from build123d import *

# Parameters (mm, degrees)
EXTRUDE_1_DEPTH          = 40
SKETCH_2_R               = 13
CUT_EXTRUDE_1_DEPTH      = 1.5
SKETCH_3_R               = 13
CUT_EXTRUDE_2_DEPTH      = 50.862310416
CUT_EXTRUDE_3_REACH      = 52.319
SKETCH_4_R               = 2
PATTERN_CIRCULAR_1_COUNT = 4
SKETCH_5_R               = 1.5
CUT_EXTRUDE_4_DEPTH      = 49.744230428
SKETCH_6_W               = 33
SKETCH_6_H               = 40
CUT_EXTRUDE_5_DEPTH      = 1.5
SKETCH_7_W               = 6
SKETCH_7_H               = 40
CUT_EXTRUDE_6_DEPTH      = 2
EXTRUDE_2_DEPTH          = 5
SKETCH_9_W               = 33
SKETCH_9_H               = 4
EXTRUDE_3_DEPTH          = 12.5
SKETCH_10_R              = 1.6
CUT_EXTRUDE_7_DEPTH      = 4
CUT_EXTRUDE_START        = -3
SKETCH_11_R              = 3
SKETCH_11_R_2            = 1.6
CUT_EXTRUDE_8_DEPTH      = 3
SKETCH_12_R              = 3
CUT_EXTRUDE_9_DEPTH      = 14


with BuildPart() as part:
    # 草图1 → 凸台-拉伸1 (new body)
    with BuildSketch(Plane.XY):
        Polygon((-16.5, 27.398785639), (-16.5, 16.398785639), (16.5, 16.398785639), (16.5, 27.398785639), (26, 27.398785639), (26, 21.398785639), (20, 21.398785639), (20, 16.398785639), (20, 11.398785639), (-20, 11.398785639), (-20, 21.398785639), (-26, 21.398785639), (-26, 27.398785639), align=None)
    extrude(amount=EXTRUDE_1_DEPTH)

    # 草图2 → 切除-拉伸1 (cut)
    with BuildSketch(Plane.XZ.offset(-11.398785639)):
        with Locations(Location((0, 20, 0), (0, 0, 270))):
            Circle(SKETCH_2_R)
    extrude(amount=-CUT_EXTRUDE_1_DEPTH, mode=Mode.SUBTRACT)

    # 草图3 → 切除-拉伸2 (cut, through all)
    with BuildSketch(Plane.XZ.offset(-12.898785639)):
        with Locations(Location((0, 20, 0), (0, 0, 270))):
            Circle(SKETCH_3_R)
    extrude(amount=-CUT_EXTRUDE_2_DEPTH, mode=Mode.SUBTRACT)

    # 草图4 → 切除-拉伸3 (cut, up to next)
    with BuildSketch(Plane.XZ.offset(-11.398785639), mode=Mode.PRIVATE) as cut_extrude_3_sk1:
        with Locations(Location((12.374368671, 32.374368671, 0), (0, 0, 270))):
            Circle(SKETCH_4_R)
    cut_extrude_3_tool1 = extrude(cut_extrude_3_sk1.sketch, amount=-CUT_EXTRUDE_3_REACH, mode=Mode.PRIVATE) & part.part
    cut_extrude_3 = cut_extrude_3_tool1.solids().sort_by_distance((12.374369, 11.398786, 32.374369))[0]
    add(cut_extrude_3, mode=Mode.SUBTRACT)

    # 阵列(圆周)1: 切除-拉伸3 ×4 about axis
    pattern_circular_1_axis = Axis((0, 0, 20), (0, 1, 0))
    for i in range(1, PATTERN_CIRCULAR_1_COUNT):
        add(cut_extrude_3.rotate(pattern_circular_1_axis, i * 360 / PATTERN_CIRCULAR_1_COUNT), mode=Mode.SUBTRACT)

    # 草图5 → 切除-拉伸4 (cut, through all)
    with BuildSketch(Plane.XZ.offset(-21.398785639)):
        with Locations(Location((-23, 27.5, 0), (0, 0, 270))):
            Circle(SKETCH_5_R)
        with Locations(Location((-23, 12.5, 0), (0, 0, 270))):
            Circle(SKETCH_5_R)
    cut_extrude_4 = extrude(amount=-CUT_EXTRUDE_4_DEPTH, mode=Mode.SUBTRACT)

    # 镜向1: 切除-拉伸4 across plane
    add(cut_extrude_4.mirror(Plane.ZY), mode=Mode.SUBTRACT)

    # 草图6 → 切除-拉伸5 (cut)
    with BuildSketch(Plane(origin=(0, 16.398785639, 0), x_dir=(1, 0, 0), z_dir=(0, 1, 0))):
        with Locations((0, -20)):
            Rectangle(SKETCH_6_W, SKETCH_6_H)
    extrude(amount=-CUT_EXTRUDE_5_DEPTH, mode=Mode.SUBTRACT)

    # 草图7 → 切除-拉伸6 (cut)
    with BuildSketch(Plane.XZ.offset(-21.398785639)):
        with Locations((-23, 20)):
            Rectangle(SKETCH_7_W, SKETCH_7_H)
        with Locations((23, 20)):
            Rectangle(SKETCH_7_W, SKETCH_7_H)
    extrude(amount=-CUT_EXTRUDE_6_DEPTH, mode=Mode.SUBTRACT)

    # 草图8 → 凸台-拉伸2 (add)
    with BuildSketch(Plane.XY):
        Polygon((20, 11.398785639), (20, 23.398785639), (26, 23.398785639), (26, 27.398785639), (16.5, 27.398785639), (16.5, 14.898785639), (-16.5, 14.898785639), (-16.5, 27.398785639), (-26, 27.398785639), (-26, 23.398785639), (-20, 23.398785639), (-20, 11.398785639), align=None)
    extrude(amount=-EXTRUDE_2_DEPTH)

    # 草图9 → 凸台-拉伸3 (add)
    with BuildSketch(Plane(origin=(0, 14.898785639, 0), x_dir=(1, 0, 0), z_dir=(0, 1, 0))):
        with Locations((0, 3)):
            Rectangle(SKETCH_9_W, SKETCH_9_H)
    extrude(amount=EXTRUDE_3_DEPTH)

    # 草图10 → 切除-拉伸7 (cut)
    with BuildSketch(Plane(origin=(0, 0, -5), x_dir=(-1, 0, 0), z_dir=(0, 0, -1))):
        with Locations((-11, 23.398785639)):
            Circle(SKETCH_10_R)
        with Locations((0, 17.398785639)):
            Circle(SKETCH_10_R)
        with Locations((11, 23.398785639)):
            Circle(SKETCH_10_R)
    extrude(amount=-CUT_EXTRUDE_7_DEPTH, mode=Mode.SUBTRACT)

    # 草图11 → 切除-拉伸8 (cut)
    # profile 1 of 3: a face of its own
    with BuildSketch(Plane.XY.offset(-1).offset(CUT_EXTRUDE_START)):
        with Locations((-11, 23.398785639)):
            Circle(SKETCH_11_R)
        with Locations(Location((-11, 23.398785639, 0), (0, 0, 180))):
            Circle(SKETCH_11_R_2, mode=Mode.SUBTRACT)
    # profile 2 of 3: a face of its own
    with BuildSketch(Plane.XY.offset(-1).offset(CUT_EXTRUDE_START)):
        with Locations((0, 17.398785639)):
            Circle(SKETCH_11_R)
        with Locations(Location((0, 17.398785639, 0), (0, 0, 180))):
            Circle(SKETCH_11_R_2, mode=Mode.SUBTRACT)
    # profile 3 of 3: a face of its own
    with BuildSketch(Plane.XY.offset(-1).offset(CUT_EXTRUDE_START)):
        with Locations((11, 23.398785639)):
            Circle(SKETCH_11_R)
        with Locations(Location((11, 23.398785639, 0), (0, 0, 180))):
            Circle(SKETCH_11_R_2, mode=Mode.SUBTRACT)
    extrude(amount=CUT_EXTRUDE_8_DEPTH, mode=Mode.SUBTRACT)

    # 草图12 → 切除-拉伸9 (cut)
    with BuildSketch(Plane.XY.offset(-1)):
        with Locations((0, 17.398785639)):
            Circle(SKETCH_12_R)
    extrude(amount=CUT_EXTRUDE_9_DEPTH, mode=Mode.SUBTRACT)


solid = part.part
Input: part model. Units: mm. Frame: model coordinates. A direction names the side the tool comes from. Give positions to 0.01 mm unless a question says otherwise; leave off trailing zeros. Write each loop counter-clockwise with the first axis right and the second up, starting at its lowest first coordinate (ties: lowest second). Pieces come first, ordered by that corner, then holes. Notation, with made-up numbers: M 2.5,49.5 L 53.5,49.5 A35 cw 53.5,83.5 Z; hole C 25,63 d1. An arc over 180 degrees is marked long. Use one line per item in the form item = value.
1. Reachability of faces 1 (the face through (12.3, 22.1, -4)), 2 (the face through (20, 17, 18)), 3 (the face through (-20, 17, 18)), 4 (the face through (-16.5, 21, 20)) from +Z, -Z, +X, -X, +Y, -Y: full face, straight path, thin tool, end or side. Return the list, or none.
Outcome:
face_1 = +Z
face_2 = +Z, -Z, +X, -Y
face_3 = +Z, -Z, -X, -Y
face_4 = +Z, +Y
2. Cut plane A-A on z = 20. Return loops of the section in (x, y), and give its area (4 significant figures).
Outcome:
outline = M -26,23.4 L -20,23.4 L -20,11.4 L -13,11.4 L -13,14.9 L -16.5,14.9 L -16.5,27.4 L -26,27.4 Z; M 13,11.4 L 20,11.4 L 20,23.4 L 26,23.4 L 26,27.4 L 16.5,27.4 L 16.5,14.9 L 13,14.9 Z
area = 184.5 mm²
3. Ray query, L1, parallel to X at y = 25.8, z = 27.5; L2, parallel to X at y = 26.5, z = 22; L3, parallel to X at y = 15.25, z = 12. Return the intervals inside material, ascending.
Outcome:
L1 = -26 to -24.5, -21.5 to -16.5, 16.5 to 21.5, 24.5 to 26
L2 = -26 to -16.5, 16.5 to 26
L3 = -20 to -16.5, 16.5 to 20
4. Mould query, pull axis Y, two halves, no side actions, for faces 5 (the face through (0, 27.399, -3)), 6 (the face through (8.6, 21.6, -2.5)), 7 (the face through (0, 21, -1)). Classes: released by +Y, released by -Y, zero draft, split by the parting line, or undercut.
Outcome:
face_5 = released by +Y
face_6 = undercut
face_7 = zero draft
5. Cut plane B-B on x = 23. Return loops of the section in (y, z), and give its area (3 significant figures).
Outcome:
outline = M 23.4,-5 L 27.4,-5 L 27.4,11 L 23.4,11 Z; M 23.4,14 L 27.4,14 L 27.4,26 L 23.4,26 Z; M 23.4,29 L 27.4,29 L 27.4,40 L 23.4,40 Z
area = 156 mm²
6. First-contact query: P1, Ø1.8, axis at x = -11.5, y = 22, coming from the +Z side; P2, Ø5, axis at y = 16, z = 6, coming from the -X side; P3, Ø1.8, axis at x = 22.5, z = 11, coming from the -Y side. Flat tips, straight axial feed; report the tip coordinate or a pass-through.
Outcome:
P1 = -4
P2 = -20
P3 = 23.4
7. Cut plane D-D on z = 1. Return loops of the section in (x, y), and give its area (3 significant figures).
Outcome:
outline = M -26,23.4 L -20,23.4 L -20,11.4 L 20,11.4 L 20,23.4 L 26,23.4 L 26,27.4 L 16.5,27.4 L 16.5,14.9 L 1.66,14.9 A3 cw -1.66,14.9 L -16.5,14.9 L -16.5,27.4 L -26,27.4 Z
area = 274 mm²
8. Cut plane C-C on x = -11. Return loops of the section in (y, z).
Outcome:
outline = M 11.4,-5 L 21.8,-5 L 21.8,-4 L 20.4,-4 L 20.4,-1 L 14.9,-1 L 14.9,6.17 L 11.4,6.17 Z; M 11.4,9.08 L 14.9,9.08 L 14.9,13.07 L 11.4,13.07 Z; M 11.4,26.93 L 14.9,26.93 L 14.9,30.92 L 11.4,30.92 Z; M 11.4,33.83 L 14.9,33.83 L 14.9,40 L 11.4,40 Z; M 25,-5 L 27.4,-5 L 27.4,-1 L 26.4,-1 L 26.4,-4 L 25,-4 Z
